from build123d import *

# Parameters (mm, degrees)
SKETCH_1_R      = 1.75
EXTRUDE_1_DEPTH = 3


with BuildPart() as part:
    # Эскиз1 → Бобышка-Вытянуть1 (new body)
    with BuildSketch(Plane.XY):
        with BuildLine():
            Line((-51.035533906, 31.464466094), (-46.464466094, 36.035533906))
            ThreePointArc((-46.464466094, 36.035533906), (-44.84234935, 37.119397663), (-42.928932188, 37.5))
            Line((-42.928932188, 37.5), (42.928932188, 37.5))
            ThreePointArc((42.928932188, 37.5), (44.84234935, 37.119397663), (46.464466094, 36.035533906))
            Line((46.464466094, 36.035533906), (51.035533906, 31.464466094))
            ThreePointArc((51.035533906, 31.464466094), (52.119397663, 29.84234935), (52.5, 27.928932188))
            Line((52.5, 27.928932188), (52.5, -27.928932188))
            ThreePointArc((52.5, -27.928932188), (52.119397663, -29.84234935), (51.035533906, -31.464466094))
            Line((51.035533906, -31.464466094), (46.464466094, -36.035533906))
            ThreePointArc((46.464466094, -36.035533906), (44.84234935, -37.119397663), (42.928932188, -37.5))
            Line((42.928932188, -37.5), (-42.928932188, -37.5))
            ThreePointArc((-42.928932188, -37.5), (-44.84234935, -37.119397663), (-46.464466094, -36.035533906))
            Line((-46.464466094, -36.035533906), (-51.035533906, -31.464466094))
            ThreePointArc((-51.035533906, -31.464466094), (-52.119397663, -29.84234935), (-52.5, -27.928932188))
            Line((-52.5, -27.928932188), (-52.5, 27.928932188))
            ThreePointArc((-52.5, 27.928932188), (-52.119397663, 29.84234935), (-51.035533906, 31.464466094))
        make_face()
        with Locations((-45.214466094, 30.214466094)):
            Circle(SKETCH_1_R, mode=Mode.SUBTRACT)
        with Locations(Location((-45.214466094, -30.214466094, 0), (0, 0, 180))):
            Circle(SKETCH_1_R, mode=Mode.SUBTRACT)
        with Locations((45.214466094, -30.214466094)):
            Circle(SKETCH_1_R, mode=Mode.SUBTRACT)
        with Locations(Location((45.214466094, 30.214466094, 0), (0, 0, 180))):
            Circle(SKETCH_1_R, mode=Mode.SUBTRACT)
    extrude(amount=EXTRUDE_1_DEPTH)


solid = part.part
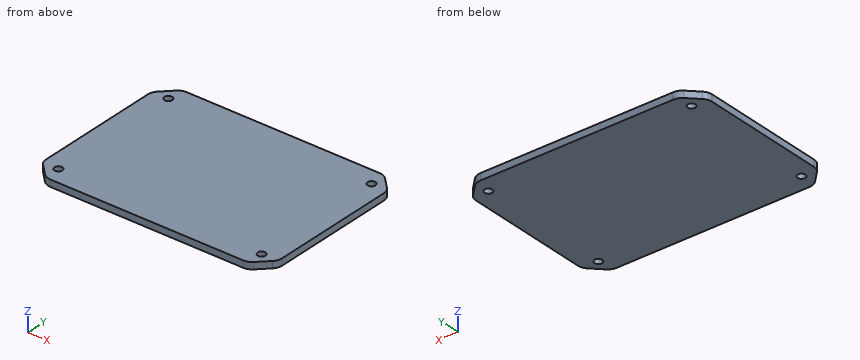
Here's how the part is built. I have some questions about the finished solid (model axes, mm). Give positions to 0.01 mm unless a question says otherwise; leave off trailing zeros. Order: outer loops, then holes, each group sorted by start corner. A loop starts at its lowest first (then second) coordinate and runs counter-clockwise, first axis right, second up. Notation, with made-up numbers: (-39.75, 1.5) -> (-7.75, 1.5) arc R26 ccw to (-7.75, 28.5) -> close; hole circle Ø8 at (3.25, 85.25). An arc over 180 degrees is marked (long way). Use a Markdown table: item, result. Add a question column.
Item 1: Will this pin go through, and if not, where does the flat tip stop? pin 1 (2 mm diameter, centred on x = 45.21, y = 30.21, fed in from +Z).
Item 2: Imagine slicing it at A-A on z = 1.5. Please give me the cut outline in (x, y).
Item 3: I need wall thicknesses on line 1 (X direction, y = 29, z = 1.25); line 2 (Y direction, x = 47, z = 1.3); line 3 (Y direction, x = 47.5, z = 0.2). Which ranges of each line are inside material? Lowest first, please.
Data:
| question | item | result |
|---|---|---|
| 1 | pin 1 | passes through |
| 2 | outline | (-52.5, -27.93) arc R5 ccw to (-51.04, -31.46) -> (-46.46, -36.04) arc R5 ccw to (-42.93, -37.5) -> (42.93, -37.5) arc R5 ccw to (46.46, -36.04) -> (51.04, -31.46) arc R5 ccw to (52.5, -27.93) -> (52.5, 27.93) arc R5 ccw to (51.04, 31.46) -> (46.46, 36.04) arc R5 ccw to (42.93, 37.5) -> (-42.93, 37.5) arc R5 ccw to (-46.46, 36.04) -> (-51.04, 31.46) arc R5 ccw to (-52.5, 27.93) -> close; hole circle Ø3.5 at (-45.21, -30.21); hole circle Ø3.5 at (-45.21, 30.21); hole circle Ø3.5 at (45.21, -30.21); hole circle Ø3.5 at (45.21, 30.21) |
| 3 | line 1 | x = -52.38 to -46.47, -43.95 to 43.95, 46.47 to 52.38 |
| 3 | line 2 | y = -35.5 to 35.5 |
| 3 | line 3 | y = -35 to 35 |
